Can you work these out from the model? Positions are in its coordinate system, mm. Round coordinates to 2 decimals unless told otherwise and drop trailing zeros. Order: outer loops, then holes, each group sorted by start corner. A loop starts at its lowest first (then second) coordinate and runs counter-clockwise, first axis right, second up.
from build123d import *

# Parameters (mm, degrees)
F0_W     = 914.4
F0_H     = 330.2
F1_DEPTH = 6.35
F2_W     = 19.05
F2_H     = 152.4
F3_DEPTH = 12.701


# Not quite as in the source:
# - a pattern or mirror of a feature is missing from the dataset's text; its kind, count and spacing are read off the source's solid


with BuildPart() as f1:
    # F0 (on Front) → F1 (new body, symmetric)
    with BuildSketch(Plane.XZ):
        Rectangle(F0_W, F0_H)
    extrude(amount=F1_DEPTH, both=True)

    # F2 (on face) → F3 (cut, through all)
    with BuildSketch(Plane.XZ.offset(6.35)):
        with Locations((314.325, -88.9)):
            Rectangle(F2_W, F2_H)
    f3 = extrude(amount=-F3_DEPTH, mode=Mode.SUBTRACT)

    # F3_copies: F3 across plane
    add(f3.mirror(Plane(origin=(0, 0, 0), x_dir=(0, 0, -1), z_dir=(-1, 0, 0))), mode=Mode.SUBTRACT)


solid = f1.part
(1) Please list where these lines run through material, in increasing order: probe 1 along X at (y, z) = (-4, -136.5); probe 2 along Z at (x, y) = (-312, -3.75).
(2) I want a section at B-B, the plane x = 313. List the corners of the cut face in (y, z) for me.
(3) I'm going to push a flat-ended pin straight in: pin 1 Ø6.5 at (x, y) = (-310, -2) entering from -Z. Where does the tip first touch, or does it pass through?
(4) I want a section at A-A, the plane y = -0.5. List the corners of the cut face in (x, z) for me.
Ans:
1. probe 1: x = -457.2 to -323.85, -304.8 to 304.8, 323.85 to 457.2
1. probe 2: z = -12.7 to 165.1
2. outline: (-6.35, -12.7) - (6.35, -12.7) - (6.35, 165.1) - (-6.35, 165.1) - close
3. pin 1: stops at z = -12.7
4. outline: (-457.2, -165.1) - (-323.85, -165.1) - (-323.85, -12.7) - (-304.8, -12.7) - (-304.8, -165.1) - (304.8, -165.1) - (304.8, -12.7) - (323.85, -12.7) - (323.85, -165.1) - (457.2, -165.1) - (457.2, 165.1) - (-457.2, 165.1) - close
